The listing builds one solid part. Answer for the finished solid, in the listing's coordinates (mm). Face numbers are marked on the shaded views. A direction names the side the tool comes from. Round coordinates to 2 decimals unless told otherwise and drop trailing zeros. Loops run counter-clockwise (first coordinate to the right, second up) from the corner with the lowest first, then second, coordinate; pieces in that order, holes last. Notation, with made-up numbers: (-29, 78) -> (-21, 78) arc R22 cw to (-21, 84) -> close; hole circle Ø7 at (-32, 53). An arc over 180 degrees is marked (long way). Write each question's results on one line, items separated by ' | '. Start each with the question number.
(1) Straight lines are drawn through the part: probe 1 along X at (y, z) = (0.9, -15); probe 2 along Z at (x, y) = (12, 1.35); probe 3 along Y at (x, z) = (21, -15.5). For each, find the intervals that lie inside material, in ascending order.
(2) Flat-ended cylindrical pins translate along their axes: pin 1 (4.5 mm diameter, centred on y = -23, z = -15.5, fed in from +X); pin 2 (4 mm diameter, centred on x = -12, z = 15, fed in from -Y); pin 3 (2 mm diameter, centred on y = -21, z = 5, fed in from -X); pin 4 (2 mm diameter, centred on x = -12, z = -15, fed in from +Y). Find the tip coordinate at first contact, or state that the pin passes through.
(3) The part is cut by section C-C (z = 15). Determine the outline of the cut face in (x, y), plus the area to 3 significant figures.
(4) The part is cut by section D-D (y = -28.5). Determine the outline of the cut face in (x, z).
(5) The part is cut by section B-B (z = 2). Determine the outline of the cut face in (x, y).
(6) For the marked faces 1 and 2, determine the directions among +Z, -Z, +X, -X, +Y, -Y from which every point of the face is accessible in a straight line to the end or side of a thin tool.
(7) The part is cut by section A-A (x = 12). Determine the outline of the cut face in (y, z).
Autodesk Inventor part; units mm, degrees
ref_plane "YZ Plane" through (0, 0, 0) normal (1, 0, 0) x (0, 1, 0)
ref_plane "XZ Plane" through (0, 0, 0) normal (0, 1, 0) x (-1, 0, 0)
ref_plane "XY Plane" through (0, 0, 0) normal (0, 0, 1) x (1, 0, 0)
sketch "草图1" plane through (0, 0, 0) normal (0, 1, 0) x (-1, 0, 0)
  line L0 (20, 20) -> (-20, 20)
  line L1 (-20, 20) -> (-20, -20)
  line L2 (-20, -20) -> (20, -20)
  line L3 (20, -20) -> (20, 20)
  point P0 (0, 0)
  dimension "d0" = 40
  dimension "d1" = 40
extrude "拉伸1" add sketch "草图1" along normal blind 3
sketch "草图6" plane through (20, 0, 20) normal (1, 0, 0) x (0, 0, -1)
  point P0 (20, 0)
sketch "草图7" plane through (20, 0, 20) normal (1, 0, 0) x (0, 0, -1)
  line L0 (40, 3) -> (0, 3)
  line L1 (0, 0) -> (40, 0)
  line L2 (40, 0) -> (40, 3)
  line L3 (40, 3) -> (0, 3)
  line L4 (0, 3) -> (0, 0)
  point P0 (20, 0)
extrude "拉伸6" add sketch "草图7" along normal blind 3
sketch "草图8" plane through (0, 0, 0) normal (0, -1, 0) x (1, 0, 0)
  line L0 (23, -20) -> (23, 20)
  line L1 (20, 20) -> (23, 20)
  line L2 (23, 20) -> (23, -20)
  line L3 (23, -20) -> (20, -20)
  line L4 (20, -20) -> (20, 20)
  point P0 (0, 0)
extrude "拉伸7" add sketch "草图8" along normal blind 47
sketch "草图9" plane through (23, 0, 20) normal (1, 0, 0) x (0, 0, -1)
  point P0 (20, 0)
sketch "草图10" plane through (23, 0, 20) normal (1, 0, 0) x (0, 0, -1)
  circle A0 centre (35.5, -23) radius 1.8
  point P0 (20, 0)
  dimension "d20" = 3.6
extrude "拉伸8" cut sketch "草图10" against normal through all
sketch "草图11" plane through (23, 0, 20) normal (1, 0, 0) x (0, 0, -1)
  circle A0 centre (4.5, -23) radius 1.8
  point P0 (20, 0)
  dimension "d23" = 3.6
extrude "拉伸9" cut sketch "草图11" against normal through all
sketch "草图12" plane through (0, 3, 0) normal (0, 1, 0) x (1, 0, 0)
  circle A0 centre (12, 15) radius 1.8
  point P0 (0, 0)
  dimension "d26" = 3.6
extrude "拉伸10" cut sketch "草图12" against normal through all
sketch "草图13" plane through (0, 3, 0) normal (0, 1, 0) x (1, 0, 0)
  circle A0 centre (-12, 15) radius 1.8
  point P0 (0, 0)
  dimension "d29" = 3.6
extrude "拉伸11" cut sketch "草图13" against normal through all
sketch "草图14" plane through (0, 3, 0) normal (0, 1, 0) x (1, 0, 0)
  circle A0 centre (-12, -15) radius 1.8
  point P0 (0, 0)
  dimension "d32" = 3.6
extrude "拉伸12" cut sketch "草图14" against normal through all
sketch "草图15" plane through (0, 3, 0) normal (0, 1, 0) x (1, 0, 0)
  circle A0 centre (12, -15) radius 1.8
  point P0 (0, 0)
  dimension "d35" = 3.6
extrude "拉伸13" cut sketch "草图15" against normal through all
equation "\"折弯半径\" = 厚度"
equation "\"折弯释压宽度\" = 厚度"
equation "\"折弯释压深度\" = 0.5 * 厚度"
equation "\"拐角释压尺寸\" = 4 * 厚度"
equation "\"最小余量\" = 2 * 厚度"
equation "\"过渡半径\" = 折弯半径"
equation "\"Jacobi半径尺寸\" = 折弯半径"
equation "\"间隙大小\" = 厚度"
properties part number "连接架"
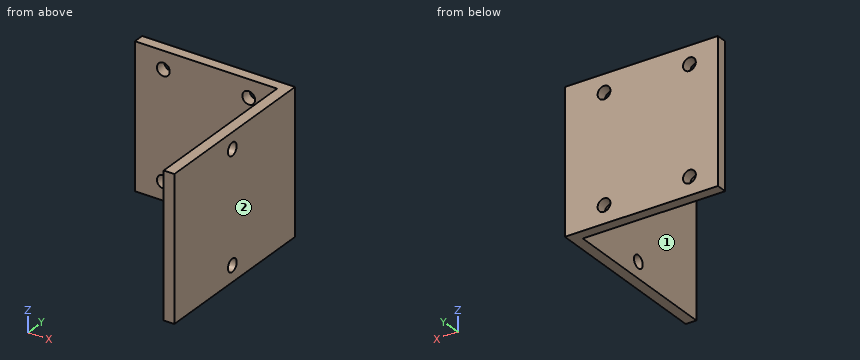
Checked values:
1) probe 1: x = -20 to -13.8, -10.2 to 10.2, 13.8 to 23 | probe 2: z = -20 to -16.8, -13.2 to 13.2, 16.8 to 20 | probe 3: y = -47 to -24.8, -21.2 to 3
2) pin 1: stops at x = 23 | pin 2: stops at y = 0 | pin 3: stops at x = 20 | pin 4: passes through
3) outline: (-20, 0) -> (-13.8, 0) -> (-13.8, 3) -> (-20, 3) -> close; (-10.2, 0) -> (10.2, 0) -> (10.2, 3) -> (-10.2, 3) -> close; (13.8, 0) -> (20, 0) -> (20, -21.27) -> (23, -21.27) -> (23, 3) -> (13.8, 3) -> close; (20, -47) -> (23, -47) -> (23, -24.73) -> (20, -24.73) -> close | area: 238 mm2
4) outline: (20, -20) -> (23, -20) -> (23, 20) -> (20, 20) -> close
5) outline: (-20, 0) -> (20, 0) -> (20, -47) -> (23, -47) -> (23, 3) -> (-20, 3) -> close
6) face 1: +Z, -Z, -X, -Y | face 2: +Z, -Z, +X, +Y, -Y
7) outline: (0, -20) -> (3, -20) -> (3, -16.8) -> (0, -16.8) -> close; (0, -13.2) -> (3, -13.2) -> (3, 13.2) -> (0, 13.2) -> close; (0, 16.8) -> (3, 16.8) -> (3, 20) -> (0, 20) -> close
